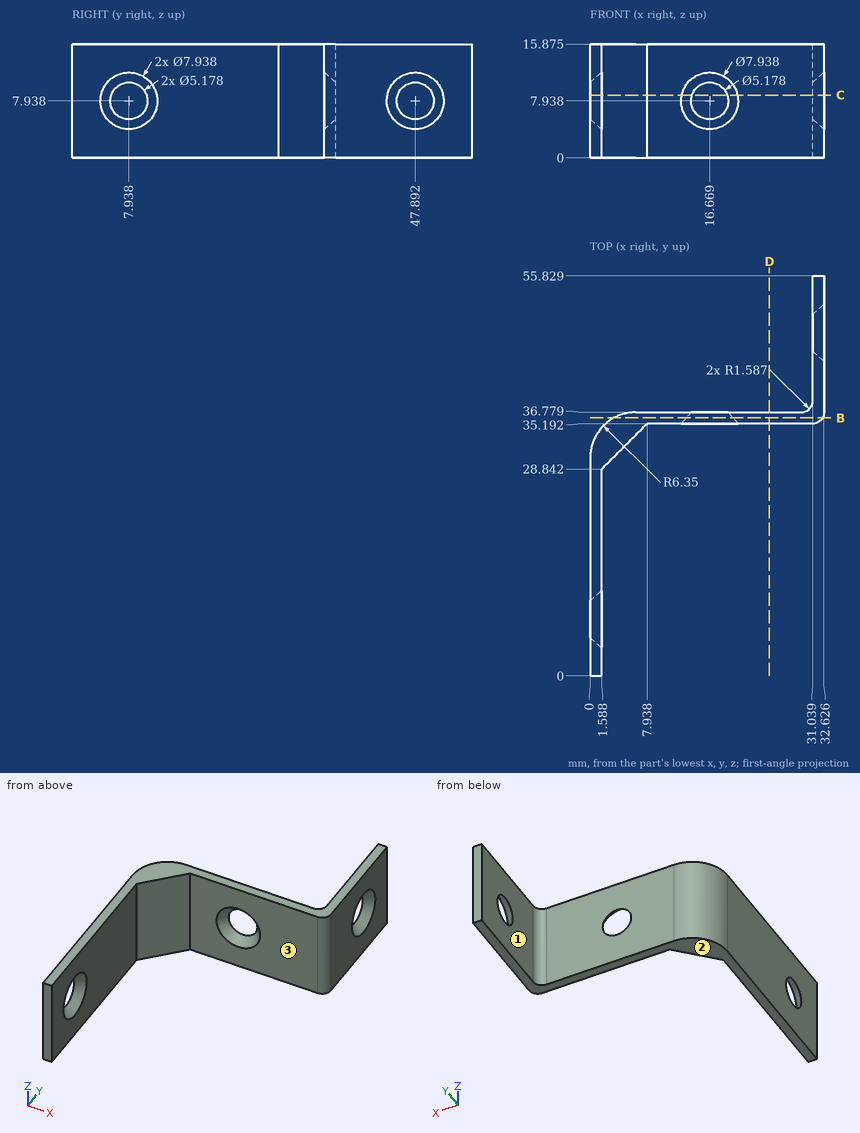
Part print with two shaded views. Sizes in mm from the minimum x, y, z corner. A direction names the side the tool comes from. Round coordinates to 2 decimals unless told otherwise and drop trailing zeros. Order: outer loops, then holes, each group sorted by start corner. A loop starts at its lowest first (then second) coordinate and runs counter-clockwise, first axis right, second up. Notation, with made-up numbers: (-1.75, 44) - (50.25, 44) arc R5 ccw to (50.25, 52) - close; hole circle Ø7 at (64, 4.5). An arc over 180 degrees is marked (long way). Answer in a Markdown table with one row per item. Add a question column.
(1) Band-saw the part on B-B on y = 36. List the corners of the cut face in (x, z) (1 decimal).
(2) Band-saw the part on D-D on x = 25. List the corners of the cut face in (y, z) (1 decimal), and give its area (3 significant figures).
(3) 3-axis set-ups, long thin cutter, end or side, ignore diameter. For the marked faces 1, 2 and 3: which of +Z, -Z, +X, -X, +Y, -Y reach the whole face in a straight line?
(4) Drop flat-ended pins along their axis: pin 1 Ø5 at (x, z) = (20, 9) entering from -Y; pin 2 Ø6 at (x, y) = (7, 34) entering from +Z (1 decimal); pin 3 Ø3 at (y, z) = (26, 4) entering from +X; pin 4 Ø2 at (x, z) = (26, 12.5) entering from +Y. Give the stop position or say it passes through.
(5) Probe L1, parallel to Y at x = 26, z = 2.5; L2, parallel to X at y = 9.5, z = 3; L3, parallel to Y at x = 13.5, z = 6.25 (1 decimal). List the from-to ranges inside material, lowest first. Write a range as [from, to].
(6) Band-saw the part on C-C on z = 8.75. Count the separate pieces of the cut face and the enclosed holes in it, and give its area (3 significant figures).
Data:
| question | item | result |
|---|---|---|
| 1 | outline | (3.3, 0) - (32.4, 0) - (32.4, 15.9) - (3.3, 15.9) - close; hole circle Ø6.5 at (16.7, 7.9) |
| 2 | outline | (35.2, 0) - (36.8, 0) - (36.8, 15.9) - (35.2, 15.9) - close |
| 2 | area | 25.2 mm^2 |
| 3 | face 1 | +Z, -Z, -X, +Y |
| 3 | face 2 | -Z, +X, -X, +Y, -Y |
| 3 | face 3 | +Z, -Z, +X, -Y |
| 4 | pin 1 | stops at y = 35.19 |
| 4 | pin 2 | stops at z = 15.9 |
| 4 | pin 3 | stops at x = 1.59 |
| 4 | pin 4 | stops at y = 36.78 |
| 5 | L1 | y = [35.19, 36.78] |
| 5 | L2 | x = [0, 1.59] |
| 5 | L3 | y = [35.6, 36.8] |
| 6 | separate pieces | 4 |
| 6 | enclosed holes | 0 |
| 6 | area | 119 mm^2 |
